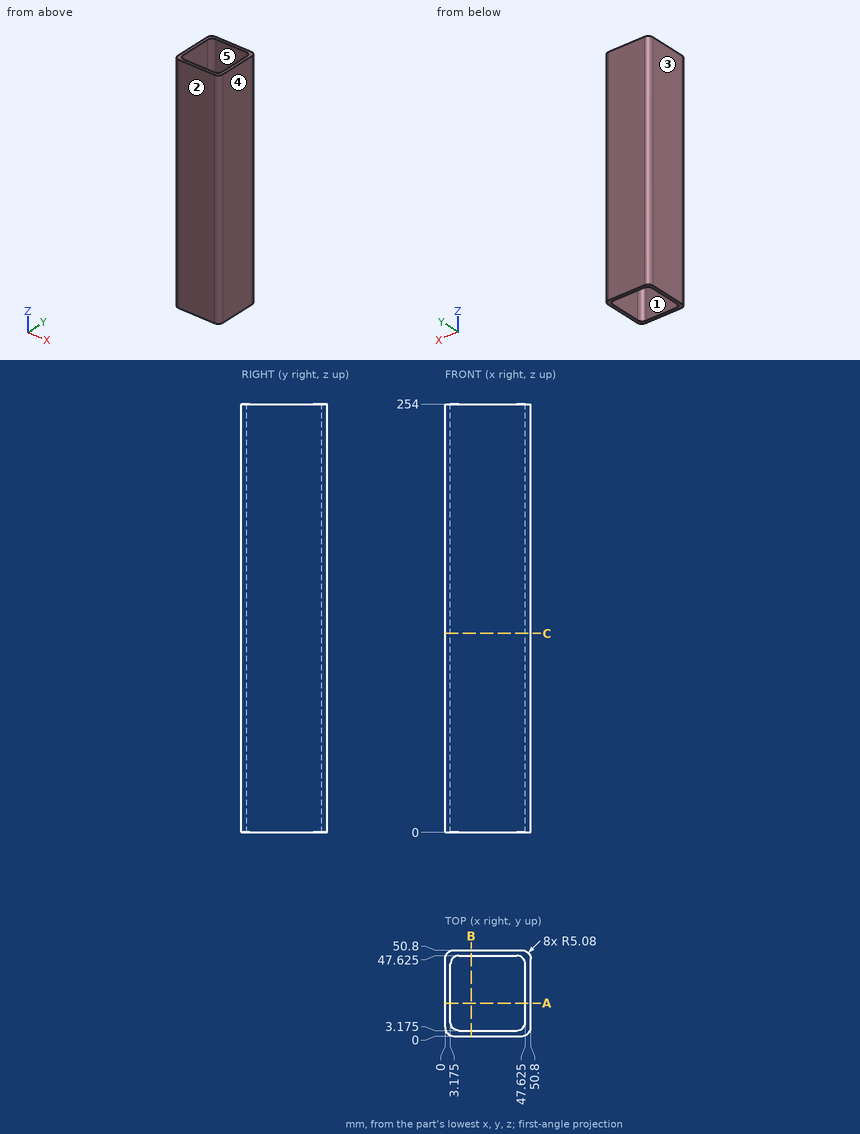
Here's the drawing with two shaded views (mm, measured from the low corner). I have some questions. A direction names the side the tool comes from. Coordinates: 2 decimals unless noted, no trailing zeros. Write each loop counter-clockwise with the first axis right and the second up, starting at its lowest first coordinate (ties: lowest second). Pieces come first, ordered by that corner, then holes. Notation, with made-up numbers: (66, -14) -> (120, -14) arc R34 ccw to (120, 19) -> close; hole circle Ø8 at (75.5, 31). An arc over 180 degrees is marked (long way). Write item = value, one per line. Start each with the question number.
(1) I need wall thicknesses on line 1 (Y direction, x = 13, z = 41.5) (3 decimals); line 2 (X direction, y = 6, z = 67). Which ranges of each line are inside material? Lowest first, please. Write a range as [from, to].
(2) Which directions (+Z, -Z, +X, -X, +Y, -Y) give clear straight access to the entire face, cutting with the end or side of a thin tool? Please do the marked faces 4 and 5.
(3) We'd pull the mould along X, two halves only. Please class the marked faces 1, 2 and 3: released by +X, released by -X, zero draft, split by the parting line, or undercut.
(4) I want a section at C-C (z = 118). Please give me the cut outline in (x, y) (3 decimals).
(5) I want a section at A-A (y = 19.5). Please give me the cut outline in (x, z) (3 decimals).
Result set:
q1.line_1 = [0, 3.175], [47.625, 50.8]
q1.line_2 = [0, 3.7], [47.1, 50.8]
q2.face_4 = +Z, -Z, +X, +Y, -Y
q2.face_5 = +Z, -Z
q3.face_1 = undercut
q3.face_2 = zero draft
q3.face_3 = released by -X
q4.outline = (0, 5.08) arc R5.08 ccw to (5.08, 0) -> (45.72, 0) arc R5.08 ccw to (50.8, 5.08) -> (50.8, 45.72) arc R5.08 ccw to (45.72, 50.8) -> (5.08, 50.8) arc R5.08 ccw to (0, 45.72) -> close; hole (3.175, 8.255) arc R5.08 ccw to (8.255, 3.175) -> (42.545, 3.175) arc R5.08 ccw to (47.625, 8.255) -> (47.625, 42.545) arc R5.08 ccw to (42.545, 47.625) -> (8.255, 47.625) arc R5.08 ccw to (3.175, 42.545) -> close
q5.outline = (0, 0) -> (3.175, 0) -> (3.175, 254) -> (0, 254) -> close; (47.625, 0) -> (50.8, 0) -> (50.8, 254) -> (47.625, 254) -> close
